```python
from build123d import *

# Parameters (mm, degrees)
F0_W     = 87.830528
F0_H     = 46.622368
F1_DEPTH = 30
F2_SIZE  = 5.08
F3_SIZE  = 10


with BuildPart() as f1:
    # F0 (on Front) → F1 (new body)
    with BuildSketch(Plane.XZ):
        with Locations((0.451185, 3.609474)):
            Rectangle(F0_W, F0_H)
    extrude(amount=F1_DEPTH)

    # F2
    f2_edges = [f1.edges().sort_by_distance(p)[0] for p in [
        (-43.464079, -30, 3.609474),
    ]]
    chamfer(f2_edges, length=F2_SIZE)

    # F3
    f3_edges = [f1.edges().sort_by_distance(p)[0] for p in [
        (2.991185, -30, 26.920658),
    ]]
    chamfer(f3_edges, length=F3_SIZE)


solid = f1.part
```
Source: CAD feature listing. Evaluate the final solid. Frame: model axes, mm. Round coordinates to 2 decimals unless told otherwise and drop trailing zeros. Write each loop counter-clockwise with the first axis right and the second up, starting at its lowest first coordinate (ties: lowest second). Pieces come first, ordered by that corner, then holes. Notation, with made-up numbers: M 18.25,35.5 L 72.25,35.5 A13 cw 72.25,57.5 Z; hole C 54,-14.5 d1. An arc over 180 degrees is marked long. Use CSV: the item, a comma, the result in double quotes. Start each with the question number.
Q1. Line query: line 1 (Y direction, x = -1, z = 17.5); line 2 (Z direction, x = -19, y = -26.75); line 3 (Y direction, x = 38, z = 24). Output: solid intervals per line, ascending. Write a range as from..to.
Q2. Cut plane A-A on x = -28.5. Output: boundary loops of the cut face in (y, z).
Q3. Cut plane B-B on y = -27. Output: boundary loops of the cut face in (x, z), plus the area to 3 significant figures.
Q4. First-contact query: P1, Ø8, axis at x = 9.5, z = 19, coming from the +Y side; P2, Ø1.5, axis at x = -14.5, y = -22, coming from the +Z side. Flat tips, straight axial feed; report the tip coordinate or a pass-through.
Q5. Cut plane C-C on z = 24.5. Output: boundary loops of the cut face in (x, y), plus the area to 3 significant figures.
Results found:
1,line 1,"-29.42..0"
1,line 2,"-19.7..20.17"
1,line 3,"-22.92..0"
2,outline,"M -30,-19.7 L 0,-19.7 L 0,26.92 L -20,26.92 L -30,16.92 Z"
3,outline,"M -41.38,-19.7 L 44.37,-19.7 L 44.37,19.92 L -41.38,19.92 Z"
3,area,"3,400 mm^2"
4,P1,"y = 0"
4,P2,"z = 25.67"
5,outline,"M -43.46,-22.42 L 44.37,-22.42 L 44.37,0 L -43.46,0 Z"
5,area,"1,970 mm^2"
